Work out the finished part from the listing and answer in its coordinate system (mm). Face numbers are marked on the shaded views. A direction names the side the tool comes from. Round coordinates to 2 decimals unless told otherwise and drop trailing zeros. Write each loop counter-clockwise with the first axis right and the second up, starting at its lowest first coordinate (ties: lowest second). Pieces come first, ordered by that corner, then holes. Notation, with made-up numbers: M 24.25,-3 L 55.25,-3 A13 cw 55.25,13 Z; hole C 75,68 d9. An arc over 180 degrees is marked long. Answer in a Markdown table with one row per item.
```python
from build123d import *

# Parameters (mm, degrees)
F0_W     = 76.2
F0_H     = 76.2
F0_W_2   = 25.4
F0_H_2   = 25.4
F0_R     = 9.525
F1_DEPTH = 6.35
F2_W     = 76.2
F2_H     = 76.2
F3_DEPTH = 6.35
F4_DEPTH = 6.35
F5_R     = 3.17499


# Not quite as in the source:
# - a fillet or chamfer is up to 0.001 mm smaller than in the source, because OpenCascade refuses the exact size


with BuildPart() as f1:
    # F0 (on Front) → F1 (new body)
    with BuildSketch(Plane.XZ):
        Rectangle(F0_W, F0_H)
        with Locations((0, -18.9619082958)):
            Rectangle(F0_W_2, F0_H_2, mode=Mode.SUBTRACT)
        with Locations((-17.78, 17.78)):
            Circle(F0_R, mode=Mode.SUBTRACT)
        Polygon((15.5130978999, 1.7698944463), (6.1174177746, 25.3682247894), (31.2520114013, 21.7059572922), align=None, mode=Mode.SUBTRACT)
    extrude(amount=-F1_DEPTH)

    # F2 (on face) → F3 (join)
    with BuildSketch(Plane.XY.offset(38.1)):
        with Locations((0, 44.45)):
            Rectangle(F2_W, F2_H)
        Polygon((-27.94, 67.8998719395), (-27.94, 72.39), (-23.4498719395, 72.39), (27.94, 72.39), (27.94, 21.0001280605), (27.94, 16.51), (23.4498719395, 16.51), (-27.94, 16.51), align=None, mode=Mode.SUBTRACT)
    extrude(amount=-F3_DEPTH)

    # F2 (on face) → F4 (join)
    with BuildSketch(Plane.XY.offset(38.1)):
        Polygon((-23.4498719395, 72.39), (-27.94, 72.39), (-27.94, 67.8998719395), (23.4498719395, 16.51), (27.94, 16.51), (27.94, 21.0001280605), align=None)
    extrude(amount=-F4_DEPTH)

    # F5 (radius 3.175 in the source; OpenCascade refuses exactly that, so slightly less here)
    f5_edges = [f1.edges().sort_by_distance(p)[0] for p in [
        (2.245064, 46.695064, 38.1),
        (-2.245064, 42.204936, 38.1),
        (-2.245064, 42.204936, 31.75),
        (2.245064, 46.695064, 31.75),
    ]]
    fillet(f5_edges, radius=F5_R)


solid = f1.part
```
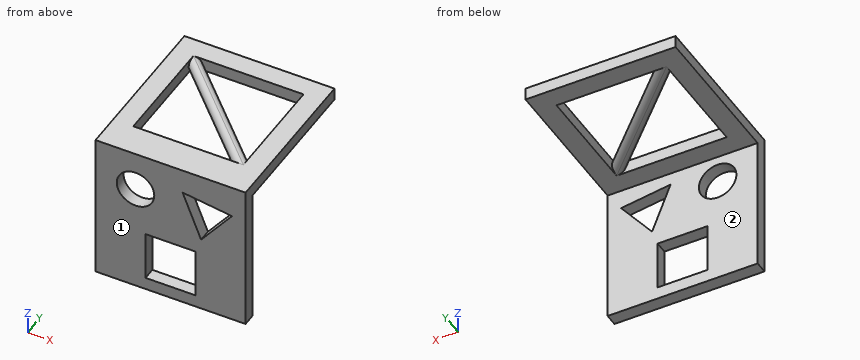
1. The part is cut by section A-A (z = -26.5). Determine the outline of the cut face in (x, y), plus the area to 3 significant figures.
Calculated:
| item | result |
|---|---|
| outline | M -38.1,0 L -12.7,0 L -12.7,6.35 L -38.1,6.35 Z; M 12.7,0 L 38.1,0 L 38.1,6.35 L 12.7,6.35 Z |
| area | 323 mm² |
2. Consider line 1 along Z through (x, y) = (-17.78, 1.5) (3 decimals); line 2 along Y through (x, z) = (4, 32.5); line 3 along X through (y, z) = (4, 17). Determine where each line is inside the solid, lowest interval first. Write a range as from..to.
Calculated:
| item | result |
|---|---|
| line 1 | z = -38.1..8.255, 27.305..38.1 |
| line 2 | y = 0..16.51, 37.55..43.35, 72.39..82.55 |
| line 3 | x = -38.1..-27.27, -8.29..9.45, 27.54..38.1 |
3. A tool of negligible diameter and unlimited length cuts with its end or side. For the marked faces 1 and 2, from which of +Z, -Z, +X, -X, +Y, -Y can it reach the whole face along a straight path? Write none if from no direction.
Calculated:
| item | result |
|---|---|
| face 1 | +Z, -Z, +X, -X, -Y |
| face 2 | -Z, +X, -X, +Y |
4. The part is cut by section C-C (x = -17). Count the separate pieces of the cut face and the enclosed holes in it, plus the area to 3 significant figures.
Calculated:
| item | result |
|---|---|
| separate pieces | 4 |
| enclosed holes | 0 |
| area | 537 mm² |
5. The part is cut by section B-B (z = 17.78). Determine the outline of the cut face in (x, y) (3 decimals).
Calculated:
| item | result |
|---|---|
| outline | M -38.1,0 L -27.305,0 L -27.305,6.35 L -38.1,6.35 Z; M -8.255,0 L 9.139,0 L 9.139,6.35 L -8.255,6.35 Z; M 28.153,0 L 38.1,0 L 38.1,6.35 L 28.153,6.35 Z |
6. Given pin 1 (10 mm diameter, centred on x = -2, z = 23.5, fed in from +Y); pin 2 (10 mm diameter, centred on x = -3, z = 13, fed in from +Y); pin 3 (6 mm diameter, centred on x = 15.5, y = 37, fed in from +Z), each flat-ended and moving along its own axis, determine where each tip first touches the part or whether it passes through.
Calculated:
| item | result |
|---|---|
| pin 1 | stops at y = 6.35 |
| pin 2 | stops at y = 6.35 |
| pin 3 | stops at z = 36.61 |
